from build123d import *

# Parameters (mm, degrees)
F0_W     = 5.55625
F0_H     = 5.55625
F0_R     = 1.5875
F1_DEPTH = 3.175
F2_R     = 1.5875
F3_DEPTH = 0.79375


with BuildPart() as f1:
    # F0 (on Front) → F1 (new body)
    with BuildSketch(Plane.XZ):
        Rectangle(F0_W, F0_H)
        Circle(F0_R, mode=Mode.SUBTRACT)
        Circle(F0_R)
    extrude(amount=F1_DEPTH)

    # F2 (on face) → F3 (join)
    with BuildSketch(Plane.XZ.offset(3.175)):
        Circle(F2_R)
    extrude(amount=F3_DEPTH)


solid = f1.part
Verification items for the finished model (mm, model axes). A direction names the side the tool comes from. Give positions to 0.01 mm unless a question says otherwise; leave off trailing zeros. Write each loop counter-clockwise with the first axis right and the second up, starting at its lowest first coordinate (ties: lowest second). Pieces come first, ordered by that corner, then holes. Notation, with made-up numbers: M 53.25,-22.75 L 66.25,-22.75 A19 cw 66.25,-5.75 Z; hole C -23.5,31.5 d7. An arc over 180 degrees is marked long. Write item = value, one per line.
(1) Access from +Z, -Z, +X, -X, +Y, -Y to the whole of each face (thin tool, end or side, straight path). Record for faces 1 (the face through (0, -2, 2.778)), 2 (the face through (-0.34, -3.57, -1.55)).
Found:
face_1 = +Z, +X, -X, +Y, -Y
face_2 = -Y
(2) Sectioned sample at D-D (x = -2). Record the cut outline in (y, z) (3 decimals).
Found:
outline = M -3.175,-2.778 L 0,-2.778 L 0,2.778 L -3.175,2.778 Z
(3) Sectioned sample at C-C (y = -3.65). Record the cut outline in (x, z) (1 decimal).
Found:
outline = C 0,0 d3.2
(4) Sectioned sample at B-B (x = 0). Record the cut outline in (y, z) (1 decimal).
Found:
outline = M -4,-1.6 L -3.2,-1.6 L -3.2,-2.8 L 0,-2.8 L 0,2.8 L -3.2,2.8 L -3.2,1.6 L -4,1.6 Z
(5) Material ranges on line 1 (Y direction, x = 0.8, z = -2.45) (3 decimals); line 2 (Z direction, x = -0.75, y = -3.8); line 3 (Z direction, x = -1.1, y = -3.5), recorded low to high.
Found:
line_1 = -3.175 to 0
line_2 = -1.4 to 1.4
line_3 = -1.14 to 1.14
(6) Sectioned sample at A-A (z = 0). Record the cut outline in (x, y) (1 decimal), then the cut area to 3 significant figures.
Found:
outline = M -2.8,-3.2 L -1.6,-3.2 L -1.6,-4 L 1.6,-4 L 1.6,-3.2 L 2.8,-3.2 L 2.8,0 L -2.8,0 Z
area = 20.2 mm2
